Drawing for the job (mm, zero at the part's lowest x, y, z). A direction names the side the tool comes from. Round coordinates to 2 decimals unless told otherwise and drop trailing zeros. Write each loop counter-clockwise with the first axis right and the second up, starting at its lowest first coordinate (ties: lowest second). Pieces come first, ordered by that corner, then holes. Notation, with made-up numbers: M -33.5,32.25 L 10.5,32.25 A20 cw 10.5,67.25 Z; hole C -16,43 d1. An arc over 180 degrees is marked long. Use a Markdown table: item, result. Add a question column.
1) Drop flat-ended pins along their axis: P1, Ø1.5, axis at x = 22, y = 37, coming from the +Z side; P2, Ø2, axis at y = 46, z = 50, coming from the -X side; P3, Ø7, axis at x = 9.1, y = 64.76, coming from the +Z side. Give the stop position or say it passes through.
2) Slice it at B-B on z = 35. Write the cut outline in (x, y), plus the area to 3 significant figures.
3) Slice it at A-A on y = 15.24. Write the cut outline in (x, z), plus the area to 3 significant figures.
4) Slice it at D-D on z = 19.5. Write the cut outline in (x, y).
5) Slice it at C-C on y = 40. Write the cut outline in (x, z).
6) Which spindle directions (+Z, -Z, +X, -X, +Y, -Y) get a long thin tool onto all of the face, cutting with end or side? Do the marked faces 4 and 5. Say none if no direction does.
7) Two-plate mould, pull along Y, no slides. Class the marked faces 1, 2 and 3: released by +Y, released by -Y, zero draft, split by the parting line, or undercut.
8) Wall check: probe 1 along Z at (x, y) = (26.5, 17); probe 2 along X at (y, z) = (64, 8) (3 decimals); probe 3 along X at (y, z) = (76.5, 41.5). Give the ranges that are in metal, low to high.
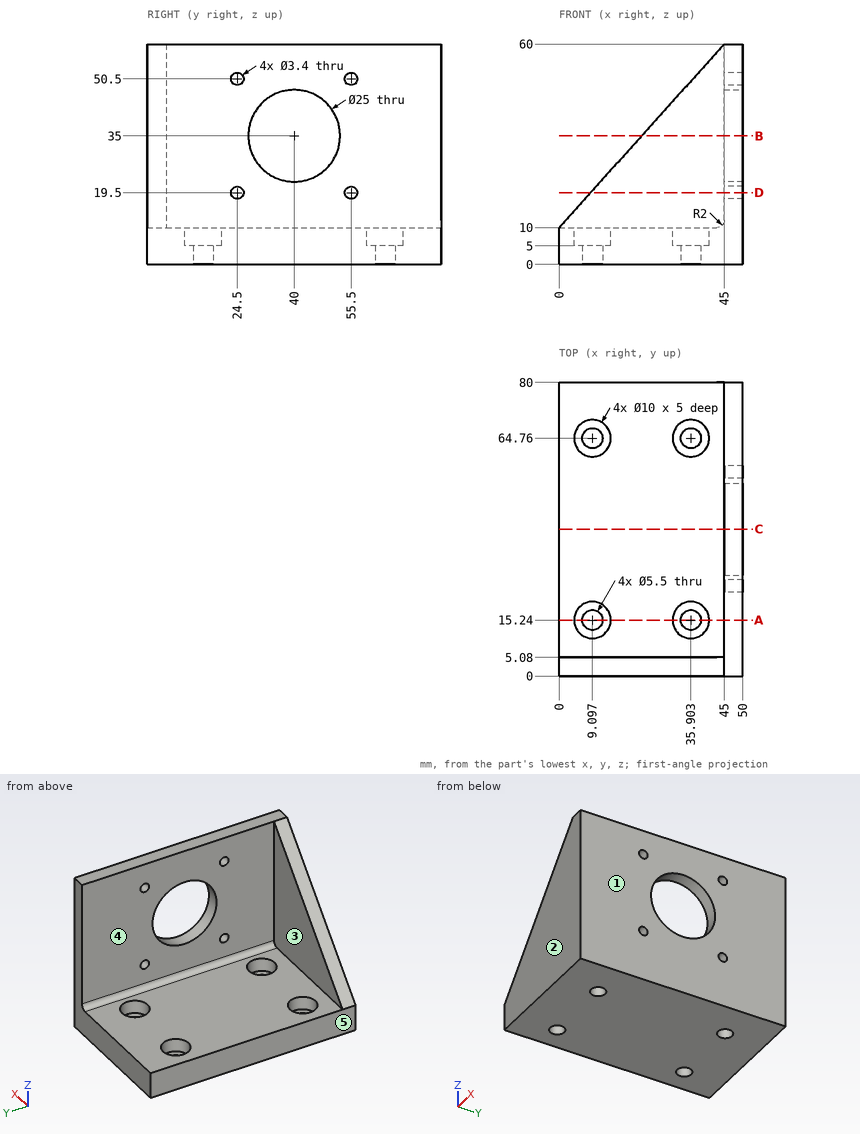
Entries:
| question | item | result |
|---|---|---|
| 1 | P1 | stops at z = 10 |
| 1 | P2 | stops at x = 45 |
| 1 | P3 | stops at z = 5 |
| 2 | outline | M 22.5,0 L 50,0 L 50,27.5 L 45,27.5 L 45,5.08 L 22.5,5.08 Z; M 45,52.5 L 50,52.5 L 50,80 L 45,80 Z |
| 2 | area | 389 mm^2 |
| 3 | outline | M 0,0 L 6.35,0 L 6.35,5 L 4.1,5 L 4.1,10 L 0,10 Z; M 11.85,0 L 33.15,0 L 33.15,5 L 30.9,5 L 30.9,10 L 14.1,10 L 14.1,5 L 11.85,5 Z; M 38.65,0 L 50,0 L 50,60 L 45,60 L 45,12 A2 cw 43,10 L 40.9,10 L 40.9,5 L 38.65,5 Z |
| 3 | area | 596 mm^2 |
| 4 | outline | M 8.55,0 L 50,0 L 50,22.8 L 45,22.8 L 45,5.08 L 8.55,5.08 Z; M 45,26.2 L 50,26.2 L 50,53.8 L 45,53.8 Z; M 45,57.2 L 50,57.2 L 50,80 L 45,80 Z |
| 5 | outline | M 0,0 L 50,0 L 50,22.5 L 45,22.5 L 45,12 A2 cw 43,10 L 0,10 Z; M 45,47.5 L 50,47.5 L 50,60 L 45,60 Z |
| 6 | face 4 | +Z, -X, +Y |
| 6 | face 5 | +Z, -Z, -X, +Y, -Y |
| 7 | face 1 | zero draft |
| 7 | face 2 | released by -Y |
| 7 | face 3 | released by +Y |
| 8 | probe 1 | z = 0 to 10 |
| 8 | probe 2 | x = 0 to 4.155, 14.039 to 30.961, 40.845 to 50 |
| 8 | probe 3 | x = 45 to 50 |
